The listing builds one solid part. Answer for the finished solid, in the listing's coordinates (mm). A direction names the side the tool comes from. Give positions to 0.01 mm unless a question says otherwise; leave off trailing zeros. Order: outer loops, then holes, each group sorted by start corner. A loop starts at its lowest first (then second) coordinate and runs counter-clockwise, first axis right, second up. Notation, with made-up numbers: M 59,60 L 70,60 A11 cw 70,65 Z; hole C -26.5,20.5 d9. An arc over 180 degrees is marked long. Answer as a JSON object with one key per item and string values. Group by question number.
```python
from build123d import *

# Parameters (mm, degrees)
BOSS_EXTRUDE1_START           = -40
BOSS_EXTRUDE1_DEPTH           = 41
SKETCH7_W                     = 1.6
SKETCH7_H                     = 83.5
M3_CLEARANCE_HOLE1_AT_2_COUNT = 2
M3_CLEARANCE_HOLE1_AT_2_PITCH = 20.75
M3_CLEARANCE_HOLE1_AT_3_COUNT = 2
M3_CLEARANCE_HOLE1_AT_3_PITCH = 35.940054257
M3_CLEARANCE_HOLE1_AT_4_COUNT = 2
M3_CLEARANCE_HOLE1_AT_4_PITCH = 41.5
M3_CLEARANCE_HOLE1_AT_5_COUNT = 2
M3_CLEARANCE_HOLE1_AT_5_PITCH = 35.940054257
M3_CLEARANCE_HOLE1_AT_6_COUNT = 2
M3_CLEARANCE_HOLE1_AT_6_PITCH = 20.75
M3_TAPPED_HOLE2_AT_2_COUNT    = 2
M3_TAPPED_HOLE2_AT_2_PITCH    = 20.75
M3_TAPPED_HOLE2_AT_3_COUNT    = 2
M3_TAPPED_HOLE2_AT_3_PITCH    = 35.940054257
M3_TAPPED_HOLE2_AT_4_COUNT    = 2
M3_TAPPED_HOLE2_AT_4_PITCH    = 41.5
M3_TAPPED_HOLE2_AT_5_COUNT    = 2
M3_TAPPED_HOLE2_AT_5_PITCH    = 35.940054257
M3_TAPPED_HOLE2_AT_6_COUNT    = 2
M3_TAPPED_HOLE2_AT_6_PITCH    = 20.75
M3_TAPPED_HOLE1_AT_2_COUNT    = 2
M3_TAPPED_HOLE1_AT_2_PITCH    = 35.940054257
M3_TAPPED_HOLE1_AT_3_COUNT    = 2
M3_TAPPED_HOLE1_AT_3_PITCH    = 35.940054257
M3_TAPPED_HOLE1_AT_4_COUNT    = 2
M3_TAPPED_HOLE1_AT_4_PITCH    = 41.401555851
M3_TAPPED_HOLE1_AT_5_COUNT    = 2
M3_TAPPED_HOLE1_AT_5_PITCH    = 41.401555851
FILLET1_R                     = 8
BOSS_EXTRUDE2_START           = 1
SKETCH18_R                    = 17.5
SKETCH18_R_2                  = 16.5
BOSS_EXTRUDE2_DEPTH           = 1
ADVANCEDHOLE1_START           = -7.819805153
ADVANCEDHOLE1_DEPTH           = 2.897488682
ADVANCEDHOLE1_START_2         = -11.819805153
ADVANCEDHOLE1_2_OUTLINE_R     = 2.15
ADVANCEDHOLE1_2_DEPTH         = 4
ADVANCEDHOLE2_START           = 4.922316471
ADVANCEDHOLE2_DEPTH           = 2.897488682
ADVANCEDHOLE2_START_2         = 7.819805153
ADVANCEDHOLE2_2_OUTLINE_R     = 2.15
ADVANCEDHOLE2_2_DEPTH         = 4
FILLET2_R                     = 0.4
FILLET4_R                     = 0.15
CHAMFER1_SIZE                 = 0.5
CHAMFER2_SIZE                 = 0.6
FILLET5_R                     = 0.4


with BuildPart() as part:
    # Sketch2 → Revolve1 (revolve)
    with BuildSketch(Plane(origin=(0, 0, 0), x_dir=(0, 0, -1), z_dir=(1, 0, 0)), mode=Mode.PRIVATE) as revolve1_sk:
        Polygon((18.5, -83.5), (18.5, -74.5), (19, -74.5), (19, -14.5), (18.5, -14.5), (18.5, -5.5), (16.5, -5.5), (16.5, -3.5), (23, -3.5), (23, -84.5), (18.5, -84.5), align=None)
    revolve(revolve1_sk.sketch.rotate(Axis((0, 55, 0), (0, -1, 0)), 180), axis=Axis((0, 55, 0), (0, -1, 0)))

    # Sketch3 → Boss-Extrude1 (add, through all)
    with BuildSketch(Plane(origin=(0, -3.5, 0), x_dir=(1, 0, 0), z_dir=(0, 1, 0)).offset(BOSS_EXTRUDE1_START)):
        with BuildLine():
            Line((-18.5, -35.215728753), (-20.621320344, -33.094408409))
            Line((-20.621320344, -33.094408409), (-14, -18.248287591))
            ThreePointArc((-14, -18.248287591), (0, -23), (14, -18.248287591))
            Line((14, -18.248287591), (20.621320344, -33.094408409))
            Line((20.621320344, -33.094408409), (18.5, -35.215728753))
            Line((18.5, -35.215728753), (9.784271247, -26.5))
            Line((9.784271247, -26.5), (9.784271247, -23.5))
            Line((9.784271247, -23.5), (-9.784271247, -23.5))
            Line((-9.784271247, -23.5), (-9.784271247, -26.5))
            Line((-9.784271247, -26.5), (-18.5, -35.215728753))
        make_face()
    extrude(amount=-BOSS_EXTRUDE1_DEPTH)

    # Sketch10 → M3 Tapped Hole2 (revolve, cut)
    with BuildSketch(Plane(origin=(0, -84.5, -20.75), x_dir=(0, 0, -1), z_dir=(1, 0, 0))):
        Polygon((0, 0), (0, 9.251075774), (1.25, 8.5), (1.25, 0), align=None)
    m3_tapped_hole2 = revolve(axis=Axis((0, -90.85, -20.75), (0, 1, 0)), mode=Mode.SUBTRACT)

    # M3 Tapped Hole2 at 2: M3 Tapped Hole2 ×2
    with Locations(*[Vector(-0.8660254037844387, 0, 0.4999999999999999) * (i * M3_TAPPED_HOLE2_AT_2_PITCH) for i in range(1, M3_TAPPED_HOLE2_AT_2_COUNT)]):
        add(m3_tapped_hole2, mode=Mode.SUBTRACT)

    # M3 Tapped Hole2 at 3: M3 Tapped Hole2 ×2
    with Locations(*[Vector(-0.5000000000000002, 0, 0.8660254037844386) * (i * M3_TAPPED_HOLE2_AT_3_PITCH) for i in range(1, M3_TAPPED_HOLE2_AT_3_COUNT)]):
        add(m3_tapped_hole2, mode=Mode.SUBTRACT)

    # M3 Tapped Hole2 at 4: M3 Tapped Hole2 ×2
    with Locations(*[(0, 0, i * M3_TAPPED_HOLE2_AT_4_PITCH) for i in range(1, M3_TAPPED_HOLE2_AT_4_COUNT)]):
        add(m3_tapped_hole2, mode=Mode.SUBTRACT)

    # M3 Tapped Hole2 at 5: M3 Tapped Hole2 ×2
    with Locations(*[Vector(0.49999999999999983, 0, 0.8660254037844388) * (i * M3_TAPPED_HOLE2_AT_5_PITCH) for i in range(1, M3_TAPPED_HOLE2_AT_5_COUNT)]):
        add(m3_tapped_hole2, mode=Mode.SUBTRACT)

    # M3 Tapped Hole2 at 6: M3 Tapped Hole2 ×2
    with Locations(*[Vector(0.8660254037844387, 0, 0.49999999999999983) * (i * M3_TAPPED_HOLE2_AT_6_PITCH) for i in range(1, M3_TAPPED_HOLE2_AT_6_COUNT)]):
        add(m3_tapped_hole2, mode=Mode.SUBTRACT)

    # Sketch15 → M3 Tapped Hole1 (revolve, cut)
    with BuildSketch(Plane(origin=(13.337842901, -3.5, -15.895422195), x_dir=(0, 0, 1), z_dir=(1, 0, 0))):
        Polygon((0, 0), (0, 8.251075774), (1.25, 7.5), (1.25, 0), align=None)
    m3_tapped_hole1 = revolve(axis=Axis((13.337842901, 2.85, -15.895422195), (0, -1, 0)), mode=Mode.SUBTRACT)

    # M3 Tapped Hole1 at 2: M3 Tapped Hole1 ×2
    with Locations(*[Vector(-0.1736481776669317, 0, 0.9848077530122079) * (i * M3_TAPPED_HOLE1_AT_2_PITCH) for i in range(1, M3_TAPPED_HOLE1_AT_2_COUNT)]):
        add(m3_tapped_hole1, mode=Mode.SUBTRACT)

    # M3 Tapped Hole1 at 3: M3 Tapped Hole1 ×2
    with Locations(*[Vector(-0.9396926207859091, 0, 0.34202014332566705) * (i * M3_TAPPED_HOLE1_AT_3_PITCH) for i in range(1, M3_TAPPED_HOLE1_AT_3_COUNT)]):
        add(m3_tapped_hole1, mode=Mode.SUBTRACT)

    # M3 Tapped Hole1 at 4: M3 Tapped Hole1 ×2
    with Locations(*[Vector(-0.6939957840318893, 0, 0.7199790634080712) * (i * M3_TAPPED_HOLE1_AT_4_PITCH) for i in range(1, M3_TAPPED_HOLE1_AT_4_COUNT)]):
        add(m3_tapped_hole1, mode=Mode.SUBTRACT)

    # M3 Tapped Hole1 at 5: M3 Tapped Hole1 ×2
    with Locations(*[Vector(-0.5885298604450689, 0, 0.8084754809915435) * (i * M3_TAPPED_HOLE1_AT_5_PITCH) for i in range(1, M3_TAPPED_HOLE1_AT_5_COUNT)]):
        add(m3_tapped_hole1, mode=Mode.SUBTRACT)

    # Fillet1
    fillet1_edges = [part.edges().sort_by_distance(p)[0] for p in [
        (-14, -64, 18.248287591),
        (14, -64, 18.248287591),
    ]]
    fillet(fillet1_edges, radius=FILLET1_R)

    # Sketch18 → Boss-Extrude2 (add)
    with BuildSketch(Plane(origin=(0, -3.5, 0), x_dir=(1, 0, 0), z_dir=(0, 1, 0)).offset(BOSS_EXTRUDE2_START)):
        with Locations(Location((0, 0, 0), (0, 0, 90))):
            Circle(SKETCH18_R)
        with Locations(Location((0, 0, 0), (0, 0, 270))):
            Circle(SKETCH18_R_2, mode=Mode.SUBTRACT)
    extrude(amount=-BOSS_EXTRUDE2_DEPTH)

    # AdvancedHole1: read off the stored shape, not the designer's step
    # AdvancedHole1 outline → AdvancedHole1 (cut)
    with BuildSketch(Plane(origin=(0, 0, 0), x_dir=(0.707106781186546, 0, 0.707106781186549), z_dir=(0.707106781186549, 0, -0.707106781186546)).offset(ADVANCEDHOLE1_START)):
        with BuildLine():
            ThreePointArc((35.372669499, 76.337703714), (27.819805153, 74.5), (35.372669499, 72.662296286))
            Line((35.372669499, 72.662296286), (36.323213796, 74.5))
            Line((36.323213796, 74.5), (35.372669499, 76.337703714))
        make_face()
        with BuildLine():
            Line((35.372669499, 51.662296286), (36.323213796, 53.5))
            Line((36.323213796, 53.5), (35.372669499, 55.337703714))
            ThreePointArc((35.372669499, 55.337703714), (27.819805153, 53.5), (35.372669499, 51.662296286))
        make_face()
    extrude(amount=ADVANCEDHOLE1_DEPTH, mode=Mode.SUBTRACT)

    # AdvancedHole1 2 outline → AdvancedHole1 2 (cut)
    with BuildSketch(Plane(origin=(0, 0, 0), x_dir=(0.707106781186546, 0, 0.707106781186549), z_dir=(0.707106781186549, 0, -0.707106781186546)).offset(ADVANCEDHOLE1_START_2)):
        with Locations((31.819805153, 74.5)):
            Circle(ADVANCEDHOLE1_2_OUTLINE_R)
        with Locations((31.819805153, 53.5)):
            Circle(ADVANCEDHOLE1_2_OUTLINE_R)
    extrude(amount=ADVANCEDHOLE1_2_DEPTH, mode=Mode.SUBTRACT)

    # AdvancedHole2: read off the stored shape, not the designer's step
    # AdvancedHole2 outline → AdvancedHole2 (cut)
    with BuildSketch(Plane(origin=(0, 0, 0), x_dir=(0.707106781186546, 0, -0.707106781186549), z_dir=(0.707106781186549, 0, 0.707106781186546)).offset(ADVANCEDHOLE2_START)):
        with BuildLine():
            Line((-36.323213796, -74.5), (-35.372669499, -76.337703714))
            ThreePointArc((-35.372669499, -76.337703714), (-27.819805153, -74.5), (-35.372669499, -72.662296286))
            Line((-35.372669499, -72.662296286), (-36.323213796, -74.5))
        make_face()
        with BuildLine():
            Line((-35.372669499, -51.662296286), (-36.323213796, -53.5))
            Line((-36.323213796, -53.5), (-35.372669499, -55.337703714))
            ThreePointArc((-35.372669499, -55.337703714), (-27.819805153, -53.5), (-35.372669499, -51.662296286))
        make_face()
    extrude(amount=ADVANCEDHOLE2_DEPTH, mode=Mode.SUBTRACT)

    # AdvancedHole2 2 outline → AdvancedHole2 2 (cut)
    with BuildSketch(Plane(origin=(0, 0, 0), x_dir=(0.707106781186546, 0, -0.707106781186549), z_dir=(0.707106781186549, 0, 0.707106781186546)).offset(ADVANCEDHOLE2_START_2)):
        with Locations((-31.819805153, -74.5)):
            Circle(ADVANCEDHOLE2_2_OUTLINE_R)
        with Locations((-31.819805153, -53.5)):
            Circle(ADVANCEDHOLE2_2_OUTLINE_R)
    extrude(amount=ADVANCEDHOLE2_2_DEPTH, mode=Mode.SUBTRACT)

    # Fillet2
    fillet2_edges = [part.edges().sort_by_distance(p)[0] for p in [
        (0, -3.5, 17.5),
    ]]
    fillet(fillet2_edges, radius=FILLET2_R)

    # Fillet4
    fillet4_edges = [part.edges().sort_by_distance(p)[0] for p in [
        (0, -5.5, -18.5),
    ]]
    fillet(fillet4_edges, radius=FILLET4_R)

    # Chamfer1
    chamfer1_edges = [part.edges().sort_by_distance(p)[0] for p in [
        (0, -14.5, -19),
        (0, -74.5, -19),
    ]]
    chamfer(chamfer1_edges, length=CHAMFER1_SIZE - 0.0001)  # a hair under: the kernel refuses the full size

    # Chamfer2
    chamfer2_edges = [part.edges().sort_by_distance(p)[0] for p in [
        (0, -84.5, -18.5),
    ]]
    chamfer(chamfer2_edges, length=CHAMFER2_SIZE)


with BuildPart() as body_2:
    # Sketch5 → Revolve2 (revolve)
    with BuildSketch(Plane(origin=(0, 0, 0), x_dir=(0, 0, -1), z_dir=(1, 0, 0)), mode=Mode.PRIVATE) as revolve2_sk:
        Polygon((18.5, -83.5), (16.5, -83.5), (16.5, -87), (23, -87), (23, -85), (18.5, -85), align=None)
    revolve(revolve2_sk.sketch.rotate(Axis((0, 55, 0), (0, -1, 0)), 180), axis=Axis((0, 55, 0), (0, -1, 0)))

    # Sketch7 → M3 Clearance Hole1 (revolve, cut)
    with BuildSketch(Plane(origin=(17.970027129, -87, -10.375), x_dir=(0, 0, -1), z_dir=(1, 0, 0))):
        with Locations((0.8, 41.75)):
            Rectangle(SKETCH7_W, SKETCH7_H)
    m3_clearance_hole1 = revolve(axis=Axis((17.970027129, -93.35, -10.375), (0, 1, 0)), mode=Mode.SUBTRACT)

    # M3 Clearance Hole1 at 2: M3 Clearance Hole1 ×2
    with Locations(*[Vector(-0.8660254037844387, 0, -0.49999999999999983) * (i * M3_CLEARANCE_HOLE1_AT_2_PITCH) for i in range(1, M3_CLEARANCE_HOLE1_AT_2_COUNT)]):
        add(m3_clearance_hole1, mode=Mode.SUBTRACT)

    # M3 Clearance Hole1 at 3: M3 Clearance Hole1 ×2
    with Locations(*[(-i * M3_CLEARANCE_HOLE1_AT_3_PITCH, 0, 0) for i in range(1, M3_CLEARANCE_HOLE1_AT_3_COUNT)]):
        add(m3_clearance_hole1, mode=Mode.SUBTRACT)

    # M3 Clearance Hole1 at 4: M3 Clearance Hole1 ×2
    with Locations(*[Vector(-0.8660254037844387, 0, 0.5) * (i * M3_CLEARANCE_HOLE1_AT_4_PITCH) for i in range(1, M3_CLEARANCE_HOLE1_AT_4_COUNT)]):
        add(m3_clearance_hole1, mode=Mode.SUBTRACT)

    # M3 Clearance Hole1 at 5: M3 Clearance Hole1 ×2
    with Locations(*[Vector(-0.5000000000000001, 0, 0.8660254037844387) * (i * M3_CLEARANCE_HOLE1_AT_5_PITCH) for i in range(1, M3_CLEARANCE_HOLE1_AT_5_COUNT)]):
        add(m3_clearance_hole1, mode=Mode.SUBTRACT)

    # M3 Clearance Hole1 at 6: M3 Clearance Hole1 ×2
    with Locations(*[(0, 0, i * M3_CLEARANCE_HOLE1_AT_6_PITCH) for i in range(1, M3_CLEARANCE_HOLE1_AT_6_COUNT)]):
        add(m3_clearance_hole1, mode=Mode.SUBTRACT)

    # Fillet5
    fillet5_edges = [body_2.edges().sort_by_distance(p)[0] for p in [
        (0, -85, -18.5),
    ]]
    fillet(fillet5_edges, radius=FILLET5_R)


solid = part.part
```
Item 1: Flat-ended cylindrical pins translate along their axes: P1, Ø2, axis at x = 0, z = 20.75, coming from the -Y side; P2, Ø3, axis at x = 15.5, y = -31.5, coming from the +Z side; P3, Ø6, axis at x = 18, y = -38, coming from the -Z side. Find the tip coordinate at first contact, or state that the pin passes through.
Item 2: Determine the mould class of faces 4 (the conical face through (7.09, -11.62, 19.28)), 5 (the flat face through (5, -43.5, 23)), 6 (the conical face through (13.33, -11.62, -16.11)), 7 (the flat face through (18.42, -63.71, 28.16)) for opening direction X: released by +X, released by -X, zero draft, split by the parting line, or undercut.
Item 3: A tool of negligible diameter and unlimited length cuts with its end or side. For faces 1 (the cylindrical face through (-18.81, -80.31, 11.3)), 2 (the cylindrical face through (-11.083, -7.198, 16.328)), 3 (the cylindrical face through (-14.955, -53.649, 24.392)), from which of +Z, -Z, +X, -X, +Y, -Y can it reach the whole face along a straight path? Write none if from no direction.
Item 4: Consider probe 1 along Y at (x, z) = (17.5, 28); probe 2 along X at (y, z) = (-6, 1); probe 3 along Y at (x, z) = (-13, -17). Determine where each line is inside the solid, lowest interval first. Write a range as from..to.
Item 5: Section B-B (y = -36.5) is taken. Determine the outline of the cut face in (x, z).
Values found:
{
 "1": {"P1": "stops at y = -75.85", "P2": "stops at z = 18.25", "P3": "stops at z = -17.44"},
 "2": {"face 4": "undercut", "face 5": "zero draft", "face 6": "undercut", "face 7": "released by +X"},
 "3": {"face 1": "-Y", "face 2": "+Y", "face 3": "none"},
 "4": {"probe 1": "y = -84.5..-78.48, -70.52..-57.48, -49.52..-43.5", "probe 2": "x = -22.98..-18.47, 18.47..22.98", "probe 3": "y = -84.5..-3.5"},
 "5": {"outline": "C 0,0 d46; hole C 0,0 d38"}
}
